Geometry check sheet. Reference: drawing and pictorial views, mm from the part's lowest x, y, z. Round coordinates to 2 decimals unless told otherwise and drop trailing zeros. Loops run counter-clockwise (first coordinate to the right, second up) from the corner with the lowest first, then second, coordinate; pieces in that order, holes last. Notation, with made-up numbers: (1.5, 74) -> (15.5, 74) arc R25 cw to (15.5, 92) -> close; hole circle Ø11 at (30.25, 0). An arc over 180 degrees is marked (long way). Write item = value, one per line.
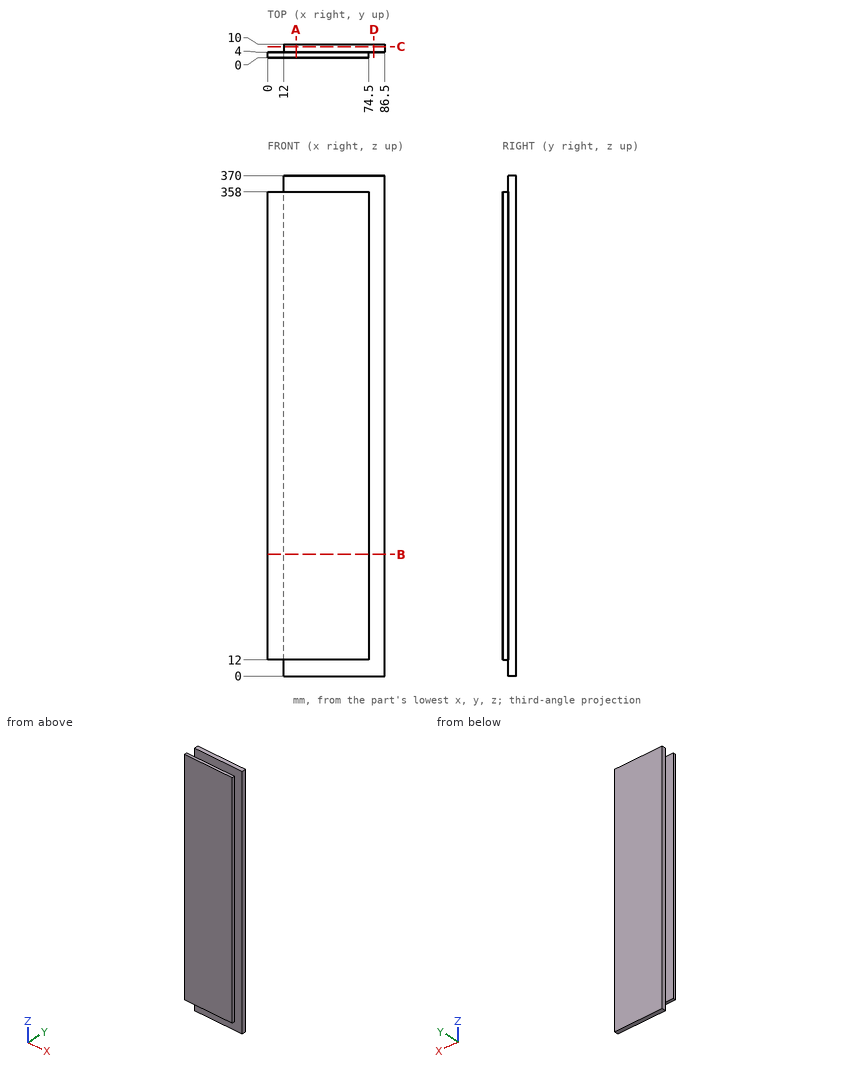
(1) Sectioned sample at C-C, the plane y = 8. Record the cut outline in (x, z).
Filled sheet:
outline = (12, 0) -> (86.5, 0) -> (86.5, 370) -> (12, 370) -> close
(2) Sectioned sample at B-B, the plane z = 90. Record the cut outline in (x, y), and give its area (3 significant figures).
Filled sheet:
outline = (0, 0) -> (74.5, 0) -> (74.5, 4) -> (86.5, 4) -> (86.5, 10) -> (12, 10) -> (12, 4) -> (0, 4) -> close
area = 745 mm2
(3) Sectioned sample at A-A, the plane x = 21. Record the cut outline in (y, z), and give its area (3 significant figures).
Filled sheet:
outline = (0, 12) -> (4, 12) -> (4, 0) -> (10, 0) -> (10, 370) -> (4, 370) -> (4, 358) -> (0, 358) -> close
area = 3,600 mm2
(4) Sectioned sample at D-D, the plane x = 78.5. Record the cut outline in (y, z), and give its area (3 significant figures).
Filled sheet:
outline = (4, 0) -> (10, 0) -> (10, 370) -> (4, 370) -> close
area = 2,220 mm2
(5) Material ranges on probe 1 along X at (y, z) = (6.5, 104.5); probe 2 along Z at (x, y) = (67, 0.5); probe 3 along X at (y, z) = (3, 40), recorded low to high. Write a range as from..to.
Filled sheet:
probe_1 = 12..86.5
probe_2 = 12..358
probe_3 = 0..74.5
(6) Go/stop test with flat-tipped pins: pin 1 Ø2 at (x, y) = (46, 2.5) entering from +Z; pin 2 Ø1.5 at (x, y) = (26.5, 3) entering from -Z; pin 3 Ø3 at (y, z) = (1.5, 146) entering from +X. Record where each tip stops, or that it passes through.
Filled sheet:
pin_1 = 358
pin_2 = 12
pin_3 = 74.5
